Can you work these out from the model? Positions are in its coordinate system, mm. Round coordinates to 2 decimals unless told otherwise and drop trailing zeros. Loops run counter-clockwise (first coordinate to the right, second up) from the corner with the lowest first, then second, coordinate; pieces in that order, holes last. Notation, with made-up numbers: (-26, 2) -> (0, 2) arc R34 cw to (0, 41) -> close; hole circle Ø11 at (-27.75, -11). An arc over 180 degrees is marked (long way). Use a Markdown table: item, result.
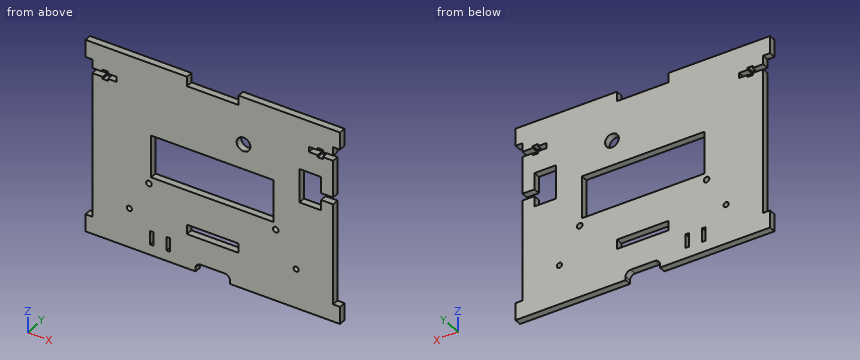
from build123d import *

# Parameters (mm, degrees)
SKETCH1_R           = 1.5
SKETCH1_R_2         = 4
SKETCH1_R_3         = 1.625
SKETCH1_W           = 30
SKETCH1_H           = 5.5
SKETCH1_W_2         = 2
SKETCH1_H_2         = 8
SKETCH1_W_3         = 71.25
SKETCH1_H_3         = 24.5
BOSS_EXTRUDE1_DEPTH = 4
FILLET1_R           = 3
FILLET2_R           = 3


with BuildPart() as part:
    # Sketch1 → Boss-Extrude1 (new body)
    with BuildSketch(Plane(origin=(0, 0, 0), x_dir=(1, 0, 0), z_dir=(0, 1, 0))):
        Polygon((85, 0), (140, 0), (144, 0), (144, 10), (140, 10), (140, 15), (134, 15), (134, 13.8), (131, 13.8), (131, 15), (126, 15), (126, 18), (131, 18), (131, 19.2), (134, 19.2), (134, 18), (140, 18), (140, 39.5), (133, 39.5), (133, 30), (120.4, 30), (120.4, 49.5), (133, 49.5), (133, 43.5), (140, 43.5), (140, 102), (144, 102), (144, 112), (140, 112), (80, 112), (80, 107), (60, 107), (60, 112), (0, 112), (-4, 112), (-4, 102), (0, 102), (0, 18), (6, 18), (6, 19.2), (9, 19.2), (9, 18), (14, 18), (14, 15), (9, 15), (9, 13.8), (6, 13.8), (6, 15), (0, 15), (0, 10), (-4, 10), (-4, 0), (0, 0), (55, 0), (55, 5.5), (85, 5.5), align=None)
        with Locations(Location((21.5, 89.25, 0), (0, 0, 270))):
            Circle(SKETCH1_R, mode=Mode.SUBTRACT)
        with Locations(Location((118.5, 89.25, 0), (0, 0, 270))):
            Circle(SKETCH1_R, mode=Mode.SUBTRACT)
        with Locations(Location((87.9, 27.5, 0), (0, 0, 270))):
            Circle(SKETCH1_R_2, mode=Mode.SUBTRACT)
        with Locations(Location((32.9, 70.5, 0), (0, 0, 270))):
            Circle(SKETCH1_R_3, mode=Mode.SUBTRACT)
        with Locations(Location((106.65, 70.5, 0), (0, 0, 270))):
            Circle(SKETCH1_R_3, mode=Mode.SUBTRACT)
        with Locations((70, 89.25)):
            Rectangle(SKETCH1_W, SKETCH1_H, mode=Mode.SUBTRACT)
        with Locations((34.5, 102)):
            Rectangle(SKETCH1_W_2, SKETCH1_H_2, mode=Mode.SUBTRACT)
        with Locations((44, 102)):
            Rectangle(SKETCH1_W_2, SKETCH1_H_2, mode=Mode.SUBTRACT)
        with Locations((69.775, 54.25)):
            Rectangle(SKETCH1_W_3, SKETCH1_H_3, mode=Mode.SUBTRACT)
    extrude(amount=BOSS_EXTRUDE1_DEPTH)

    # Fillet1
    fillet1_edges = [part.edges().sort_by_distance(p)[0] for p in [
        (60, 2, -107),
    ]]
    fillet(fillet1_edges, radius=FILLET1_R)

    # Fillet2
    fillet2_edges = [part.edges().sort_by_distance(p)[0] for p in [
        (80, 2, -107),
    ]]
    fillet(fillet2_edges, radius=FILLET2_R)


solid = part.part
1. Will these pins go through, and if not, where does the flat tip stop? pin 1 Ø0.6 at (y, z) = (3, -18.5) entering from -X; pin 2 Ø2 at (y, z) = (1, -100.5) entering from +X.
Answer sheet:
| item | result |
|---|---|
| pin 1 | stops at x = 0 |
| pin 2 | stops at x = 140 |
2. I want a section at B-B (z = -27.5). Please give me the cut outline in (x, y).
Answer sheet:
| item | result |
|---|---|
| outline | (0, 0) -> (83.9, 0) -> (83.9, 4) -> (0, 4) -> close; (91.9, 0) -> (140, 0) -> (140, 4) -> (91.9, 4) -> close |
3. I want a section at A-A (x = 118.5). Please give me the cut outline in (y, z), plus the area to 3 significant figures.
Answer sheet:
| item | result |
|---|---|
| outline | (0, -112) -> (4, -112) -> (4, -90.75) -> (0, -90.75) -> close; (0, -87.75) -> (4, -87.75) -> (4, 0) -> (0, 0) -> close |
| area | 436 mm² |
4. I need wall thicknesses on line 1 (X direction, y = 0.75, z = -100.5); line 2 (X direction, y = 1.15, z = -70.5) (3 decimals); line 3 (Z direction, x = 73, y = 2.5). Which ranges of each line are inside material? Lowest first, please.
Answer sheet:
| item | result |
|---|---|
| line 1 | x = 0 to 33.5, 35.5 to 43, 45 to 140 |
| line 2 | x = 0 to 31.275, 34.525 to 105.025, 108.275 to 140 |
| line 3 | z = -107 to -92, -86.5 to -66.5, -42 to -5.5 |
5. I want a section at D-D (y = 1.05). State how many separate pieces and enclosed holes the cut face has, plus the area to 3 significant figures.
Answer sheet:
| item | result |
|---|---|
| separate pieces | 1 |
| enclosed holes | 9 |
| area | 13,200 mm² |
6. I want a section at C-C (x = 87.9). Please give me the cut outline in (y, z), plus the area to 3 significant figures.
Answer sheet:
| item | result |
|---|---|
| outline | (0, -112) -> (4, -112) -> (4, -66.5) -> (0, -66.5) -> close; (0, -42) -> (4, -42) -> (4, -31.5) -> (0, -31.5) -> close; (0, -23.5) -> (4, -23.5) -> (4, 0) -> (0, 0) -> close |
| area | 318 mm² |
